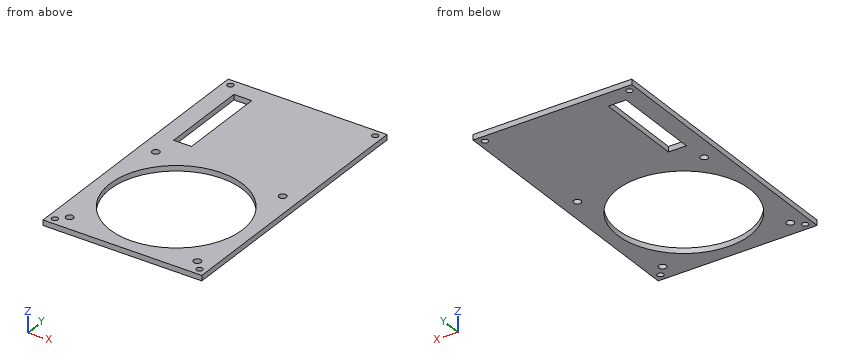
Autodesk Inventor part; units mm, degrees
ref_plane "YZ Plane" through (0, 0, 0) normal (1, 0, 0) x (0, 1, 0)
ref_plane "XZ Plane" through (0, 0, 0) normal (0, 1, 0) x (-1, 0, 0)
ref_plane "XY Plane" through (0, 0, 0) normal (0, 0, 1) x (1, 0, 0)
sketch "Boceto1" plane through (0, 0, 0) normal (0, 0, 1) x (1, 0, 0)
  line L0 (-44.66, 76.85) -> (-44.66, -76.85)
  line L1 (-44.66, -76.85) -> (44.66, -76.85)
  line L2 (44.66, -76.85) -> (44.66, 76.85)
  line L3 (44.66, 76.85) -> (-44.66, 76.85)
  line L4 (41.66, -73.85) -> (-41.66, -73.85)
  line L5 (-41.66, -73.85) -> (-41.66, 73.85)
  line L6 (-41.66, 73.85) -> (41.66, 73.85)
  line L7 (41.66, 73.85) -> (41.66, -73.85)
  point P0 (0, 0)
extrude "Extrusión1" add sketch "Boceto1" along normal blind 3 contours L3 L2 L1 L0 | L4 L5 L6 L7
sketch "Boceto2" plane through (0, 0, 3) normal (0, 0, 1) x (1, 0, 0)
  line L0 (15.66, 13.175) -> (25.66, 13.175)
  line L1 (25.66, 13.175) -> (25.66, 9.175)
  line L2 (25.66, 9.175) -> (15.66, 9.175)
  line L3 (15.66, 9.175) -> (15.66, 13.175)
  line L4 (-21.66, 30.85) -> (-31.66, 30.85)
  line L5 (-31.66, 30.85) -> (-31.66, 34.85)
  line L6 (-31.66, 34.85) -> (-21.66, 34.85)
  line L7 (-21.66, 34.85) -> (-21.66, 30.85)
  line L8 (25.66, 30.85) -> (15.66, 30.85)
  line L9 (15.66, 30.85) -> (15.66, 34.85)
  line L10 (15.66, 34.85) -> (25.66, 34.85)
  line L11 (25.66, 34.85) -> (25.66, 30.85)
  line L12 (-31.66, 13.175) -> (-21.66, 13.175)
  line L13 (-21.66, 13.175) -> (-21.66, 9.175)
  line L14 (-21.66, 9.175) -> (-31.66, 9.175)
  line L15 (-31.66, 9.175) -> (-31.66, 13.175)
  circle A0 centre (32.34, 65.85) radius 4.5
  circle A1 centre (-33.66, 39.85) radius 4.5
  line L16 (38.16, -57.55) -> (38.16, -73.85)
  line L17 (38.16, -73.85) -> (41.66, -73.85)
  line L18 (41.66, -73.85) -> (41.66, 73.85)
  line L19 (41.66, 73.85) -> (-41.66, 73.85)
  line L20 (-41.66, 73.85) -> (-41.66, -73.85)
  line L21 (-41.66, -73.85) -> (23.76, -73.85)
  circle A2 centre (32.34, 39.85) radius 4.5
  circle A3 centre (-33.66, 65.85) radius 4.5
  line L22 (-44.66, 76.85) -> (-44.66, -76.85)
  line L23 (-44.66, 76.85) -> (-44.66, -76.85)
  line L24 (-44.66, -76.85) -> (44.66, -76.85)
  line L25 (44.66, -76.85) -> (44.66, 76.85)
  line L26 (44.66, 76.85) -> (-44.66, 76.85)
  line L27 (-44.66, 76.85) -> (-44.66, -76.85)
  line L28 (-41.66, -73.85) -> (41.66, -73.85)
  line L29 (41.66, -73.85) -> (41.66, 73.85)
  line L30 (41.66, 73.85) -> (-41.66, 73.85)
  line L31 (-41.66, 73.85) -> (-41.66, -73.85)
  line L32 (-41.66, -73.85) -> (41.66, -73.85)
  line L33 (41.66, -73.85) -> (41.66, 9.47)
  line L34 (41.66, 9.47) -> (-41.66, 9.47)
  line L35 (-41.66, 9.47) -> (-41.66, -73.85)
  line L36 (40, 7.81) -> (-40, 7.81)
  line L37 (-40, 7.81) -> (-40, -72.19)
  line L38 (-40, -72.19) -> (40, -72.19)
  line L39 (40, -72.19) -> (40, 7.81)
  line L40 (40, 7.81) -> (-40, -72.19) construction
  line L41 (-40, 7.81) -> (40, -72.19) construction
  line L42 (-37.8, -69.99) -> (-37.8, 5.61)
  line L43 (-37.8, 5.61) -> (37.8, 5.61)
  line L44 (37.8, 5.61) -> (37.8, -69.99)
  line L45 (37.8, -69.99) -> (-37.8, -69.99)
  circle A4 centre (-35.7, -67.89) radius 2.1
  circle A5 centre (0, -32.19) radius 37.25
  circle A6 centre (-35.7, 3.51) radius 2.1
  circle A7 centre (35.7, 3.51) radius 2.1
  circle A8 centre (35.7, -67.3145) radius 2.1
  point P0 (0, 0)
  dimension "d9" = 83.32
  dimension "d10" = 83.32
  dimension "d11" = 83.32
  dimension "d12" = 80
  dimension "d13" = 80
  dimension "d14" = 2.2
  dimension "d15" = 4.2
  dimension "d16" = 74.5
  dimension "d17" = 4.2
  dimension "d18" = 4.2
  dimension "d19" = 4.2
extrude "Extrusión3" cut sketch "Boceto2" against normal blind 3 contours A8 | A4 | A6 | A7 | A5
sketch "Boceto4" plane through (0, 0, 3) normal (0, 0, 1) x (1, 0, 0)
  circle A0 centre (35.7, 3.51) radius 2.1
  circle A1 centre (35.7, -67.3145) radius 2.1
  circle A2 centre (-35.7, 3.51) radius 2.1
  circle A3 centre (-35.7, -67.89) radius 2.1
  circle A4 centre (0, -32.19) radius 37.25
  line L0 (-44.66, -76.85) -> (44.66, -76.85)
  line L1 (44.66, -76.85) -> (44.66, 76.85)
  line L2 (44.66, 76.85) -> (-44.66, 76.85)
  line L3 (-44.66, 76.85) -> (-44.66, -76.85)
  line L4 (-34.66, -66.85) -> (34.66, -66.85)
  line L5 (34.66, -66.85) -> (34.66, 66.85)
  line L6 (34.66, 66.85) -> (-34.66, 66.85)
  line L7 (-34.66, 66.85) -> (-34.66, -66.85)
  line L8 (-34.66, 66.85) -> (-24.66, 66.85)
  line L9 (-24.66, 66.85) -> (-24.66, 16.85)
  line L10 (-24.66, 16.85) -> (-34.66, 16.85)
  line L11 (-34.66, 16.85) -> (-34.66, 66.85)
  point P0 (0, 0)
  point P1 (-34.66, 16.85)
  dimension "d22" = 10
  dimension "d23" = 10
  dimension "d24" = 50
extrude "Extrusión4" cut sketch "Boceto4" against normal blind 10 contours L9 L10 L7 L6
sketch "Boceto5" plane through (0, 0, 0) normal (0, 0, -1) x (-1, 0, 0)
  circle A0 centre (-40.66, -72.85) radius 1.75
  circle A1 centre (40.66, -72.85) radius 1.75
  circle A2 centre (40.66, 72.85) radius 1.75
  circle A3 centre (-40.66, 72.85) radius 1.75
  point P0 (0, 0)
hole "Agujero1" at (40.66, 72.85, 0) at (-40.66, 72.85, 0) at (-40.66, -72.85, 0) at (40.66, -72.85, 0) direction (0, 0, 1) diameter 3.5 depth 7
properties part number "TapaControladora"
Geometry check sheet. Reference: the model listing, model coordinates, mm. Give positions to 0.01 mm unless a question says otherwise; leave off trailing zeros. Order: outer loops, then holes, each group sorted by start corner. A loop starts at its lowest first (then second) coordinate and runs counter-clockwise, first axis right, second up. Notation, with made-up numbers: (65, 32.5) - (70, 32.5) arc R32 ccw to (70, 65.5) - close; hole circle Ø9 at (79, 37.25). An arc over 180 degrees is marked (long way). Answer in a Markdown table with one row per item. Add a question column.
Q1. Gauge pin test, flat end, axial feed: pin 1 (3 mm diameter, centred on x = 40.66, y = 72.85, fed in from -Z). Record the tip position at first contact, or that the pin passes through.
Q2. Cross-section at C-C, the plane x = -9.5. Enter the section's corners in (y, z), then the cut area to 3 significant figures.
Q3. Material ranges on probe 1 along Y at (x, z) = (-40.66, 1.1); probe 2 along X at (y, z) = (-72.85, 1.2); probe 3 along X at (y, z) = (65.5, 1.35), recorded low to high. Write a range as from..to.
Q4. Cross-section at B-B, the plane y = 51. Enter the section's corners in (x, z).
Q5. Cross-section at D-D, the plane y = 3.51. Enter the section's corners in (x, z), then the cut area to 3 significant figures.
Q6. Cross-section at A-A, the plane x = -40.66. Enter the section's corners in (y, z).
Check values:
| question | item | result |
|---|---|---|
| 1 | pin 1 | passes through |
| 2 | outline | (-76.85, 0) - (-68.21, 0) - (-68.21, 3) - (-76.85, 3) - close; (3.83, 0) - (76.85, 0) - (76.85, 3) - (3.83, 3) - close |
| 2 | area | 245 mm^2 |
| 3 | probe 1 | y = -76.85..-74.6, -71.1..71.1, 74.6..76.85 |
| 3 | probe 2 | x = -44.66..-42.41, -38.91..38.91, 42.41..44.66 |
| 3 | probe 3 | x = -44.66..-34.66, -24.66..44.66 |
| 4 | outline | (-44.66, 0) - (-34.66, 0) - (-34.66, 3) - (-44.66, 3) - close; (-24.66, 0) - (44.66, 0) - (44.66, 3) - (-24.66, 3) - close |
| 5 | outline | (-44.66, 0) - (-37.8, 0) - (-37.8, 3) - (-44.66, 3) - close; (-33.6, 0) - (-10.63, 0) - (-10.63, 3) - (-33.6, 3) - close; (10.63, 0) - (33.6, 0) - (33.6, 3) - (10.63, 3) - close; (37.8, 0) - (44.66, 0) - (44.66, 3) - (37.8, 3) - close |
| 5 | area | 179 mm^2 |
| 6 | outline | (-76.85, 0) - (-74.6, 0) - (-74.6, 3) - (-76.85, 3) - close; (-71.1, 0) - (71.1, 0) - (71.1, 3) - (-71.1, 3) - close; (74.6, 0) - (76.85, 0) - (76.85, 3) - (74.6, 3) - close |
